Read the model definition and answer for the solid it produces. Units are mm, in the model's axes. A direction names the side the tool comes from. Coordinates: 2 decimals unless noted, no trailing zeros. Write each loop counter-clockwise with the first axis right and the second up, starting at its lowest first coordinate (ties: lowest second). Pieces come first, ordered by that corner, then holes.
(1) Determine the mould class of faces 4 (the cylindrical face through (361.399, -36.215, 549.273)), 5 (the flat face through (178.06, -238.55, 331.33)), 6 (the cylindrical face through (237.307, -96.765, 425.18)) for opening direction Y: pulls with the +Y half, pulls with the -Y half, needs draft (parallel to the pull), parting line crosses it, or undercut.
(2) Which of the six approach directions +Z, -Z, +X, -X, +Y, -Y give full straight-line access (tool end or side, diameter ignored) to faces 1 (the flat face through (626, -239, 0)), 2 (the flat face through (388.88, -240.33, 575.8)), 3 (the flat face through (904, -178.942, -24))?
(3) The part is cut by section B-B, the plane y = -270. Determine the outline of the cut face in (x, z), and give its area (3 significant figures).
(4) The part is cut by section A-A, the plane x = 834. Determine the outline of the cut face in (y, z), and give its area (3 significant figures).
(5) The part is cut by section C-C, the plane y = -451. Determine the outline of the cut face in (x, z), and give its area (3 significant figures).
(6) The part is cut by section D-D, the plane z = 129. Determine the outline of the cut face in (x, y), and give its area (3 significant figures).
(7) Given pin 1 (1 mm diameter, centred on x = 999.5, y = -423.5, fed in from +Z); pin 2 (3 mm diameter, centred on y = -318.5, z = 252.5, fed in from +X); pin 3 (6 mm diameter, centred on y = -163, z = 38, fed in from +X), each flat-ended and moving along its own axis, determine where each tip first touches the part or whether it passes through.
(8) Straight lines are drawn through the part: line 1 along Y through (x, z) = (457.2, -17) (3 decimals); line 2 along Z through (x, y) = (941.5, -360); line 3 along Z through (x, y) = (235.5, -350). For each, find the intervals that lie inside material, in ascending order.
```python
from build123d import *

# Parameters (mm, degrees)
F0_W     = 1270
F0_H     = 48.26
F1_DEPTH = 483.87
F2_R     = 63.5
F3_DEPTH = 48.261
F4_R     = 127
F5_R     = 38.1
F6_DEPTH = 1088.7905941503


with BuildPart() as f1:
    # F0 (on Front) → F1 (new body)
    with BuildSketch(Plane.XZ):
        with Locations((635, -24.13)):
            Rectangle(F0_W, F0_H)
        with BuildLine():
            Line((0, -48.26), (0, 0))
            ThreePointArc((0, 0), (-59.0920227604, 40.2369511729), (-43.3079228428, 109.9631412552))
            Line((-43.3079228428, 109.9631412552), (405.7048832106, 558.9759473086))
            Line((405.7048832106, 558.9759473086), (371.5799099506, 593.1009205687))
            Line((371.5799099506, 593.1009205687), (-77.4328961029, 144.0881145152))
            ThreePointArc((-77.4328961029, 144.0881145152), (-103.6745515501, 21.7641046473), (0, -48.26))
        make_face()
    extrude(amount=F1_DEPTH)

    # F2 (on face) → F3 (cut, through all)
    with BuildSketch(Plane.XY):
        with Locations((457.2, -241.935)):
            Circle(F2_R)
        with BuildLine():
            ThreePointArc((1092.2007215854, -305.9415523028), (1155.7007215854, -242.4415523028), (1092.2007215854, -178.9415523028))
            Line((1092.2007215854, -178.9415523028), (711.2007215854, -178.9415523028))
            ThreePointArc((711.2007215854, -178.9415523028), (647.7007215854, -242.4415523028), (711.2007215854, -305.9415523028))
            Line((711.2007215854, -305.9415523028), (1092.2007215854, -305.9415523028))
        make_face()
    extrude(amount=-F3_DEPTH, mode=Mode.SUBTRACT)

    # F4
    f4_edges = [f1.edges().sort_by_distance(p)[0] for p in [
        (388.642397, 0, 576.038434),
        (388.642397, -483.87, 576.038434),
        (1270, -483.87, -24.13),
        (1270, 0, -24.13),
    ]]
    fillet(f4_edges, radius=F4_R)

    # F5 (on face) → F6 (cut, through all)
    with BuildSketch(Plane(origin=(-110.7605053091, 0, 110.7605053091), x_dir=(0, -1, 0), z_dir=(-0.7071067812, 0, 0.7071067812))):
        with Locations((127, 491.6323569408)):
            Circle(F5_R)
        with Locations((356.87, 491.6323569408)):
            Circle(F5_R)
    extrude(amount=-F6_DEPTH, mode=Mode.SUBTRACT)


solid = f1.part
```
Computed:
1. face 4: pulls with the +Y half
1. face 5: needs draft
1. face 6: undercut
2. face 1: +X, +Y, -Y
2. face 2: +Z, +X, +Y, -Y
2. face 3: +Z, -Z
3. outline: (-77.43, 144.09) arc R111.76 ccw to (0, -48.26) - (400.24, -48.26) - (400.24, 0) - (0, 0) arc R63.51 cw to (-43.31, 109.96) - (405.7, 558.98) - (371.58, 593.1) - close; (514.16, -48.26) - (653.99, -48.26) - (653.99, 0) - (514.16, 0) - close; (1149.41, -48.26) - (1270, -48.26) - (1270, 0) - (1149.41, 0) - close
3. area: 72,600 mm2
4. outline: (-483.87, -48.26) - (-305.94, -48.26) - (-305.94, 0) - (-483.87, 0) - close; (-178.94, -48.26) - (0, -48.26) - (0, 0) - (-178.94, 0) - close
4. area: 17,200 mm2
5. outline: (-77.43, 144.09) arc R111.76 ccw to (0, -48.26) - (1228.26, -48.26) - (1228.26, 0) - (0, 0) arc R63.51 cw to (-43.31, 109.96) - (376.19, 529.46) - (342.06, 563.58) - close
5. area: 98,000 mm2
6. outline: (-90.55, -483.87) - (-24.27, -483.87) - (-24.27, 0) - (-90.55, 0) - close
6. area: 32,100 mm2
7. pin 1: stops at z = 0
7. pin 2: stops at x = 100.73
7. pin 3: stops at x = -56.75
8. line 1: y = -483.87 to -305.435, -178.435 to 0
8. line 2: z = -48.26 to 0
8. line 3: z = -48.26 to 0, 388.77 to 406.77
